```python
from build123d import *

# Parameters (mm, degrees)
SKETCH1_W           = 315.575
SKETCH1_H           = 92
SKETCH1_W_2         = 309.225
SKETCH1_H_2         = 85.65
BOSS_EXTRUDE1_DEPTH = 235.775
SKETCH1_2_W         = 309.225
SKETCH1_2_H         = 85.65
BOSS_EXTRUDE2_DEPTH = 3.175


with BuildPart() as part:
    # Sketch1 → Boss-Extrude1 (new body)
    with BuildSketch(Plane.XY):
        Rectangle(SKETCH1_W, SKETCH1_H)
        Rectangle(SKETCH1_W_2, SKETCH1_H_2, mode=Mode.SUBTRACT)
    extrude(amount=BOSS_EXTRUDE1_DEPTH)

    # Sketch1<2> → Boss-Extrude2 (add)
    with BuildSketch(Plane.XY):
        Rectangle(SKETCH1_2_W, SKETCH1_2_H)
    extrude(amount=BOSS_EXTRUDE2_DEPTH)


solid = part.part
```
Geometry: final body of the model. Coordinates: model frame, mm. A direction names the side the tool comes from. Round coordinates to 2 decimals unless told otherwise and drop trailing zeros. Write each loop counter-clockwise with the first axis right and the second up, starting at its lowest first coordinate (ties: lowest second). Pieces come first, ordered by that corner, then holes. Notation, with made-up numbers: (-34.5, -7) -> (-13.5, -7) arc R36 cw to (-13.5, 32) -> close; hole circle Ø2 at (49, 9). An arc over 180 degrees is marked (long way). Return JSON: item names as keys, results as strings.
Q1. Section A-A on y = -3. Return the cut outline in (x, z) (1 decimal).
From the geometry:
{"outline": "(-157.8, 0) -> (157.8, 0) -> (157.8, 235.8) -> (154.6, 235.8) -> (154.6, 3.2) -> (-154.6, 3.2) -> (-154.6, 235.8) -> (-157.8, 235.8) -> close"}
Q2. Section C-C on x = 108.5. Return the cut outline in (y, z) (3 decimals).
From the geometry:
{"outline": "(-46, 0) -> (46, 0) -> (46, 235.775) -> (42.825, 235.775) -> (42.825, 3.175) -> (-42.825, 3.175) -> (-42.825, 235.775) -> (-46, 235.775) -> close"}
Q3. Set-up query: faces 1 (the flat face through (-2, 1, 0)), 2 (the flat face through (-2, 1, 3.175)). Return all of +Z, -Z, +X, -X, +Y, -Y with unobstructed straight access to the full face (end or side cutting, diameter ignored); none if empty.
From the geometry:
{"face 1": "-Z, +X, -X, +Y, -Y", "face 2": "+Z"}
Q4. Ray query, line 1 (X direction, y = -13.5, z = 66); line 2 (Y direction, x = 42, z = 65.5) (3 decimals); line 3 (Z direction, x = -67, y = -17) (3 decimals). Return the intervals inside material, ascending.
From the geometry:
{"line 1": "-157.79 to -154.61, 154.61 to 157.79", "line 2": "-46 to -42.825, 42.825 to 46", "line 3": "0 to 3.175"}
Q5. Section B-B on z = 54.5. Return the cut outline in (x, y) (1 decimal), and give its area (3 significant figures).
From the geometry:
{"outline": "(-157.8, -46) -> (157.8, -46) -> (157.8, 46) -> (-157.8, 46) -> close; hole (-154.6, -42.8) -> (154.6, -42.8) -> (154.6, 42.8) -> (-154.6, 42.8) -> close", "area": "2,550 mm2"}
Q6. First-contact query: pin 1 Ø8 at (x, y) = (28, 3.5) entering from +Z (3 decimals). Flat tip, straight axial feed; report the tip coordinate or a pass-through.
From the geometry:
{"pin 1": "z = 3.175"}
